Part model, mm, in its own coordinate system. A direction names the side the tool comes from. Coordinates: 2 decimals unless noted, no trailing zeros. Loops run counter-clockwise (first coordinate to the right, second up) from the corner with the lowest first, then second, coordinate; pieces in that order, holes last. Notation, with made-up numbers: (2, 15) - (24, 15) arc R6 cw to (24, 24) - close; hole circle Ø10 at (19.5, 24.5). An arc over 180 degrees is marked (long way). Use a Markdown table: item, result. Add a question column.
1) Pull direction Y, two halves, no side cores. Call faces 1 (the face through (0, -11, 8)), 2 (the face through (8, 30, 7)), 3 (the face through (-7, 11, 0)): +Y half, -Y half, draft (parallel to the pull), parting line (faces both ways), or undercut.
2) Band-saw the part on D-D (x = 0). Give the cut face in (y, z).
3) Drop flat-ended pins along their axis: P1, Ø3, axis at x = 0, z = 9.5, coming from the +Y side; P2, Ø8, axis at y = -2.5, z = 10, coming from the -X side; P3, Ø2, axis at x = -0.5, z = 13.5, coming from the -Y side. Give the stop position or say it passes through.
4) Tool access for faces 4 (the face through (-0.391, -7.712, 4.526)), 5 (the face through (7.46, 29.4, 14.43)), 6 (the face through (-5, 14.5, 9.1)): list every direction of +Z, -Z, +X, -X, +Y, -Y with a clear straight run to the whole face (end or side of a thin tool).
5) Band-saw the part on B-B (y = 11). Give the cut face in (x, z).
6) Probe probe 1 along Z at (x, y) = (7.3, 20); probe 2 along X at (y, z) = (7, 13.75); probe 3 along Y at (x, z) = (-3, 6). List the from-to ranges inside material, lowest first. Write a range as [from, to].
7) Band-saw the part on C-C (z = 7.5). Give the number of separate pieces and of enclosed holes in the cut face, plus the area to 3 significant figures.
8) Band-saw the part on A-A (y = 20). Give the cut face in (x, z), plus the area to 3 significant figures.
Autodesk Inventor part; units mm, degrees
ref_plane "YZ Plane" through (0, 0, 0) normal (1, 0, 0) x (0, 1, 0)
ref_plane "XZ Plane" through (0, 0, 0) normal (0, 1, 0) x (-1, 0, 0)
ref_plane "XY Plane" through (0, 0, 0) normal (0, 0, 1) x (1, 0, 0)
sketch "Schizzo1" plane through (0, 0, 0) normal (0, 0, 1) x (1, 0, 0)
  line L0 (-10, 30) -> (-10, 0)
  line L1 (-10, 0) -> (10, 0)
  line L2 (10, 0) -> (10, 30)
  line L3 (10, 30) -> (5, 30)
  line L4 (5, 30) -> (5, 5)
  line L5 (5, 5) -> (-5, 5)
  line L6 (-5, 5) -> (-5, 30)
  line L7 (-5, 30) -> (-10, 30)
  point P0 (0, 0)
  point P1 (0, 5)
  point P2 (0, 0)
  dimension "d0" = 20
  dimension "d1" = 10
  dimension "d2" = 5
  dimension "d3" = 30
extrude "Estrusione1" add sketch "Schizzo1" along normal blind 15
sketch "Schizzo2" plane through (0, 0, 0) normal (1, 0, 0) x (0, 1, 0)
  line L0 (5, 0) -> (30, 0)
  line L1 (30, 0) -> (30, 15)
  line L2 (5, 15) -> (30, 15)
  line L3 (5, 0) -> (5, 15)
  circle A0 centre (20, 7.5) radius 5
  point P0 (0, 0)
  point P1 (30, 7.5)
  point P2 (17.5, 0)
  dimension "d6" = 10
  dimension "d23" = 10
extrude "Estrusione2" cut sketch "Schizzo2" along normal through all both and the other way through all contours A0
fillet "Raccordo1" radius 2 6 edges at (-7.5, 30, 15) (-7.5, 30, 0) (7.5, 30, 15) (7.5, 30, 0) (10, 0, 7.5) (-10, 0, 7.5)
sketch "Schizzo3" plane through (-8, 0, 0) normal (0, -1, 0) x (1, 0, 0)
  line L0 (0, 0) -> (0, 15)
  line L1 (0, 0) -> (16, 0)
  line L2 (16, 15) -> (16, 0)
  line L3 (0, 15) -> (16, 15)
  circle A0 centre (8, 7.5) radius 6
  point P0 (8, 0)
  point P1 (16, 7.5)
  point P2 (8, 0)
  dimension "d13" = 12
extrude "Estrusione3" add sketch "Schizzo3" along normal blind 5 contours A0
sketch "Schizzo4" plane through (0, -5, 7.5) normal (0, -1, 0) x (1, 0, 0)
  circle A0 centre (0, 0) radius 3
  point P0 (0, -7.5)
  dimension "d16" = 6
extrude "Estrusione4" add sketch "Schizzo4" along normal blind 6
chamfer "Smusso1" distance 0.5 angle 45 6 edges at (-5, 15, 7.5) (5, 15, 7.5) (-10, 15, 7.5) (10, 15, 7.5) (-3, -11, 7.5) (-6, -5, 7.5)
thread "Filettatura2"
properties part number "Forcella movimento lama" material "Acciaio inossidabile"
Answer block:
| question | item | result |
|---|---|---|
| 1 | face 1 | -Y half |
| 1 | face 2 | +Y half |
| 1 | face 3 | draft |
| 2 | outline | (-11, 5) - (-10.5, 4.5) - (-5, 4.5) - (-5, 2) - (-4.5, 1.5) - (0, 1.5) - (0, 0) - (5, 0) - (5, 15) - (0, 15) - (0, 13.5) - (-4.5, 13.5) - (-5, 13) - (-5, 10.5) - (-10.5, 10.5) - (-11, 10) - close |
| 3 | P1 | y = 5 |
| 3 | P2 | x = -9.94 |
| 3 | P3 | y = -5 |
| 4 | face 4 | -Y |
| 4 | face 5 | +Z, +X, -X, +Y |
| 4 | face 6 | +Z, -Z, +Y |
| 5 | outline | (-10, 0) - (-5, 0) - (-5, 15) - (-10, 15) - close; (5, 0) - (10, 0) - (10, 15) - (5, 15) - close |
| 6 | probe 1 | [0, 2.5], [12.5, 15] |
| 6 | probe 2 | [-10, -5], [5, 10] |
| 6 | probe 3 | [-5, 5] |
| 7 | separate pieces | 3 |
| 7 | enclosed holes | 0 |
| 7 | area | 343 mm2 |
| 8 | outline | (-10, 0) - (-5, 0) - (-5, 2) - (-5.5, 2.5) - (-9.5, 2.5) - (-10, 2) - close; (-10, 13) - (-9.5, 12.5) - (-5.5, 12.5) - (-5, 13) - (-5, 15) - (-10, 15) - close; (5, 0) - (10, 0) - (10, 2) - (9.5, 2.5) - (5.5, 2.5) - (5, 2) - close; (5, 13) - (5.5, 12.5) - (9.5, 12.5) - (10, 13) - (10, 15) - (5, 15) - close |
| 8 | area | 49.0 mm2 |
